Autodesk Inventor part; units mm, degrees
ref_plane "YZ Plane" through (0, 0, 0) normal (1, 0, 0) x (0, 1, 0)
ref_plane "XZ Plane" through (0, 0, 0) normal (0, 1, 0) x (-1, 0, 0)
ref_plane "XY Plane" through (0, 0, 0) normal (0, 0, 1) x (1, 0, 0)
sketch "Эскиз1" plane through (0, 0, 0) normal (1, 0, 0) x (0, 1, 0)
  line L0 (4.2947, -1.2) -> (3.8947, -1.2)
  line L1 (3.8947, -1.2) -> (0, -1.2)
  line L2 (0, -1.2) -> (-1, -1.2)
  line L3 (-4, 22.6194) -> (-4, -13.7271)
  line L4 (-1, -1.2) -> (-2.2, -1.2)
  line L5 (-2.2, -2.95) -> (-2.2, -1.2)
  line L6 (-2.2504, -1.2) -> (-4.2, -1.2)
  line L7 (-2.2, -1.2) -> (-2.2504, -1.2)
  line L8 (-4.2947, 1.2) -> (4.2947, 1.2)
  line L9 (4.2947, 1.2) -> (4.2947, -1.2)
  line L10 (4.2947, -1.2) -> (-4.2947, -1.2)
  line L11 (-4.2947, -1.2) -> (-4.2947, 1.2)
  line L12 (-4.2947, 1.2) -> (4.2947, -1.2) construction
  line L13 (4.2947, 1.2) -> (-4.2947, -1.2) construction
  line L14 (4.2947, -1.35) -> (-4, -0.9878)
  line L15 (4.2947, -1.35) -> (4.2947, -1.2)
  line L16 (-4, -1.2) -> (-4, -0.9878)
  line L17 (4.2947, 0) -> (-4, 0)
  line L18 (4.2947, 1.35) -> (-4, 0.9878)
  line L19 (4.2947, 1.35) -> (4.2947, 1.2)
  point P0 (0, 0)
  point P1 (-4, 0.9878)
  dimension "d0" = 2.5
  dimension "d1" = 0.15
extrude "Выдавливание1" add sketch "Эскиз1" along normal mid plane 6 contours L15 L14 L1 L0 | L0 L1 L14 L3 L17 L9 | L17 L3 L18 L8 L9 | L8 L18 L19
sketch "Эскиз2" plane through (-3, 4.2947, 1.35) normal (0, 1, 0) x (1, 0, 0)
  line L0 (5.25, 0.15) -> (0.75, 0.15)
  arc A0 (0.75, 0.15) -> (5.25, 0.15) centre (3, 1.35) ccw
  line L1 (0.75, 2.55) -> (5.25, 2.55)
  arc A1 (5.25, 2.55) -> (0.75, 2.55) centre (3, 1.35) ccw
  circle A2 centre (3, 1.35) radius 2.55
  line L2 (0, 0) -> (6, 0)
  line L3 (6, 2.7) -> (6, 0)
  line L4 (0, 2.7) -> (6, 2.7)
  line L5 (0, 0) -> (0, 2.7)
  arc A3 (5.6949, 2.55) -> (0.3051, 2.55) centre (3, 1.35) ccw
  arc A4 (0.3051, 0.15) -> (5.6949, 0.15) centre (3, 1.35) ccw
  circle A5 centre (3, 1.35) radius 2.95
  point P0 (3, 1.35)
  point P1 (0.8367, 0)
  point P2 (0.8367, 2.7)
  point P3 (5.1633, 2.7)
  point P4 (5.1633, 0)
  point P5 (5.623, 2.7)
  point P6 (5.6949, 0.15)
  point P7 (5.623, 0)
  point P8 (0.377, 0)
  point P9 (0.3051, 0.15)
  point P10 (0.3051, 2.55)
  point P11 (0.377, 2.7)
extrude "Выдавливание2" cut sketch "Эскиз2" against normal blind 10 contours A4 A5 A3 L4 L3 L2 | L2 L5 L4 A3 A5 A4
properties part number "middle_gear_vtilka_shtift"
Source: CAD feature listing. Evaluate the final solid. Frame: model axes, mm. Coordinates: 2 decimals unless noted, no trailing zeros. Loops run counter-clockwise (first coordinate to the right, second up) from the corner with the lowest first, then second, coordinate; pieces in that order, holes last. Notation, with made-up numbers: M -16.5,56 L 4.5,56 A22 ccw 4.5,92 Z; hole C 51.5,2 d10. An arc over 180 degrees is marked long. Use a Markdown table: item, result. Add a question column.
Q1. Section query B-B, the plane z = -0.55. Return loops of the section in (x, y).
Q2. Section query A-A, the plane y = 2.5. Return loops of the section in (x, z).
Q3. First-contact query: pin 1 (2 mm diameter, centred on x = 0, y = 0, fed in from +Z); pin 2 (2 mm diameter, centred on x = -2, y = 2, fed in from -Z). Flat tips, straight axial feed; report the tip coordinate or a pass-through.
Q4. Material intervals for L1, parallel to Z at x = -2.2, y = -2.5; L2, parallel to Z at x = -2.25, y = 0.75; L3, parallel to X at y = 2, z = -0.15, sorted ascending.
Q5. Section query C-C, the plane x = -0.7. Return loops of the section in (y, z), and give its area (3 significant figures).
Result:
| question | item | result |
|---|---|---|
| 1 | outline | M -2.9,-4 L 2.9,-4 L 2.9,4.29 L -2.9,4.29 Z |
| 2 | outline | M -2.69,-1.2 A2.95 ccw -2.66,-1.27 L 2.66,-1.27 A2.95 ccw 2.69,-1.2 A2.95 ccw 2.69,1.2 A2.95 ccw 2.66,1.27 L -2.66,1.27 A2.95 ccw -2.69,1.2 A2.95 ccw Z |
| 3 | pin 1 | stops at z = 1.21 |
| 3 | pin 2 | stops at z = -1.29 |
| 4 | L1 | z = -1.05 to 1.05 |
| 4 | L2 | z = -1.2 to 1.2 |
| 4 | L3 | x = -2.95 to 2.95 |
| 5 | outline | M -4,-0.99 L 4.29,-1.35 L 4.29,1.35 L -4,0.99 Z |
| 5 | area | 19.4 mm2 |
